Autodesk Inventor part; units mm, degrees
ref_plane "YZ Plane" through (0, 0, 0) normal (1, 0, 0) x (0, 1, 0)
ref_plane "XZ Plane" through (0, 0, 0) normal (0, 1, 0) x (-1, 0, 0)
ref_plane "XY Plane" through (0, 0, 0) normal (0, 0, 1) x (1, 0, 0)
sketch "Sketch1" plane through (0, 0, 0) normal (0, 0, 1) x (1, 0, 0)
  line L0 (0, 0) -> (101.6, 0)
  line L1 (101.6, 0) -> (101.6, 107.95)
  line L2 (101.6, 107.95) -> (0, 107.95)
  line L3 (0, 107.95) -> (0, 0)
  dimension "d0" = 101.6
  dimension "d1" = 107.95
extrude "Extrusion1" add sketch "Sketch1" along normal blind 6.35
sketch "Sketch2" plane through (0, 0, 6.35) normal (0, 0, 1) x (1, 0, 0)
  line L0 (101.6, 107.95) -> (0, 107.95)
  line L1 (101.6, 0) -> (101.6, 107.95)
  line L2 (0, 0) -> (101.6, 0)
  point P0 (50.8, 87.122)
  point P1 (50.8, 107.95)
  point P2 (101.6, 53.975)
  dimension "d31" = 20.828
hole "Hole1" at (50.8, 87.122, 6.35) direction (0, 0, -1) diameter 9.525 depth 19.05 tip angle 118
sketch "Sketch3" plane through (0, 0, 6.35) normal (0, 0, 1) x (1, 0, 0)
  line L0 (101.6, 107.95) -> (0, 107.95)
  line L1 (0, 107.95) -> (0, 0)
  circle A0 centre (50.8, 87.122) radius 4.7625
  point P0 (12.7, 87.122)
  point P1 (88.9, 87.122)
  dimension "d12" = 12.7
  dimension "d15" = 76.2
hole "Hole2" at (12.7, 87.122, 6.35) at (88.9, 87.122, 6.35) direction (0, 0, -1) diameter 3.175 depth 19.05 tip angle 118 counterbore diameter 6.35 counterbore depth 3.175
sketch "Sketch4" plane through (0, 0, 6.35) normal (0, 0, 1) x (1, 0, 0)
  circle A0 centre (50.8, 87.122) radius 4.7625
  point P0 (0, 0)
  point P1 (50.8, 39.122)
  dimension "d39" = 48
hole "Hole3" at (50.8, 39.122, 6.35) direction (0, 0, -1) diameter 6.35 depth 19.05 tip angle 118
sketch "Sketch6" plane through (0, 0, 0) normal (0, 0, -1) x (-1, 0, 0)
  circle A0 centre (-50.8, 87.122) radius 4.7625
  point P0 (0, 0)
  point P1 (-50.8, 101.4095)
  point P2 (-50.8, 72.8345)
  dimension "d52" = 28.575
  dimension "d53" = 14.2875
hole "Hole5" at (50.8, 101.4095, 0) at (50.8, 72.8345, 0) direction (0, 0, 1) diameter 3.81 depth 19.05 tip angle 118 counterbore diameter 6.35 counterbore depth 0.508
sketch "Sketch7" plane through (0, 0, 6.35) normal (0, 0, 1) x (1, 0, 0)
  circle A0 centre (50.8, 101.4095) radius 1.905
  circle A1 centre (50.8, 72.8345) radius 1.905
  point P0 (0, 0)
hole "Hole6" at (50.8, 101.4095, 6.35) at (50.8, 72.8345, 6.35) direction (0, 0, -1) diameter 3.81 depth 19.05 tip angle 118 counterbore diameter 7.1374 counterbore depth 3.5052
sketch "Sketch8" plane through (0, 0, 6.35) normal (0, 0, 1) x (1, 0, 0)
  circle A0 centre (50.8, 46.122) radius 15.5
  circle A1 centre (50.8, 39.122) radius 3.175
  point P0 (0, 0)
  point P1 (66.3, 46.122)
  point P2 (58.55, 59.5454)
  point P3 (43.05, 59.5454)
  point P4 (35.3, 46.122)
  point P5 (43.05, 32.6986)
  point P6 (58.55, 32.6986)
  dimension "d68" = 31
  dimension "d69" = 7
  dimension "d79" = 360
hole "Hole8" at (66.3, 46.122, 6.35) at (58.55, 59.5454, 6.35) at (43.05, 59.5454, 6.35) at (35.3, 46.122, 6.35) at (43.05, 32.6986, 6.35) at (58.55, 32.6986, 6.35) direction (0, 0, -1) diameter 3.4036 depth 12.2936 tip angle 118 counterbore diameter 6.5024 counterbore depth 2.9972
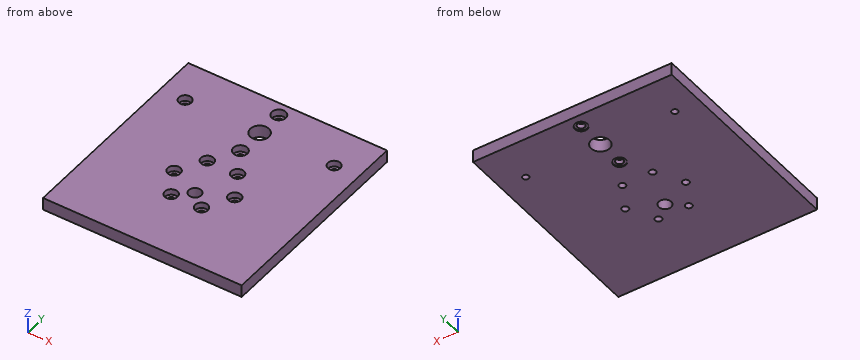
Can you work these out from the model? Positions are in its coordinate system, mm. Coordinates: 2 decimals unless noted, no trailing zeros. Order: outer loops, then holes, each group sorted by start corner. A loop starts at its lowest first (then second) coordinate and runs counter-clockwise, first axis right, second up. Notation, with made-up numbers: (14, -10) - (39, -10) arc R21 ccw to (39, 20) - close; hole circle Ø1 at (-25.75, 72). An arc over 180 degrees is marked (long way). Answer as a JSON object with one key per item and string values. Group by question number.
Q1. I need wall thicknesses on line 1 (Y direction, x = 50.8, z = 3.5); line 2 (Y direction, x = 58.55, z = 2); line 3 (Y direction, x = 66.3, z = 1.1). Which ranges of each line are inside material? Lowest first, please. Write a range as from..to.
Q2. Imagine slicing it at A-A (x = 58.55). Please give me the cut outline in (y, z).
Q3. Imagine slicing it at B-B (z = 5). Give the number of separate pieces and of enclosed holes in the cut face, and give its area (3 significant figures).
Q4. Will these pins go through, and if not, where does the flat tip stop? P1, Ø3, axis at x = 66.3, y = 46.122, coming from the -Z side; P2, Ø5, axis at x = 43.05, y = 59.55, coming from the +Z side; P3, Ø2, axis at x = 49, y = 101, coming from the +Z side.
Determined:
{
 "1": {"line 1": "y = 0..35.95, 42.3..69.27, 76.4..82.36, 91.88..97.84, 104.98..107.95", "line 2": "y = 0..31, 34.4..57.84, 61.25..107.95", "line 3": "y = 0..44.42, 47.82..107.95"},
 "2": {"outline": "(0, 0) - (31, 0) - (31, 3.35) - (29.45, 3.35) - (29.45, 6.35) - (0, 6.35) - close; (34.4, 0) - (57.84, 0) - (57.84, 3.35) - (56.29, 3.35) - (56.29, 6.35) - (35.95, 6.35) - (35.95, 3.35) - (34.4, 3.35) - close; (61.25, 0) - (107.95, 0) - (107.95, 6.35) - (62.8, 6.35) - (62.8, 3.35) - (61.25, 3.35) - close"},
 "3": {"separate pieces": "1", "enclosed holes": "12", "area": "10,500 mm2"},
 "4": {"P1": "passes through", "P2": "stops at z = 3.35", "P3": "stops at z = 2.84"}
}
